Build history of the part. All positions in model axes, mm. A direction names the side the tool comes from. Give positions to 0.01 mm unless a question says otherwise; leave off trailing zeros. Write each loop counter-clockwise with the first axis right and the second up, starting at its lowest first coordinate (ties: lowest second). Pieces come first, ordered by that corner, then holes. Notation, with made-up numbers: M 85.5,-22.5 L 89.5,-22.5 A11 ccw 89.5,-13.5 Z; hole C -19,56 d1. An arc over 180 degrees is marked long. One line per item, written item: value. Start each with the question number.
from build123d import *

# Parameters (mm, degrees)
F1_DEPTH       = 20
F2_D           = 8
F2_CBORE_D     = 12.5
F2_CBORE_DEPTH = 12.5
F3_D           = 8
F3_CBORE_D     = 12.5
F3_CBORE_DEPTH = 12.5


with BuildPart() as f1:
    # F0 (on Front) → F1 (new body)
    with BuildSketch(Plane.XZ):
        Polygon((197.0788455009, 58.5275515914), (-137.9211544991, 58.5275515914), (-137.9211544991, -121.4724484086), (-102.9211544991, -121.4724484086), (-102.9211544991, -1.4724484086), (-77.9211544991, -1.4724484086), (-77.9211544991, -121.4724484086), (-42.9211544991, -121.4724484086), (-42.9211544991, -1.4724484086), (-17.9211544991, -1.4724484086), (-17.9211544991, -121.4724484086), (17.0788455009, -121.4724484086), (17.0788455009, -1.4724484086), (42.0788455009, -1.4724484086), (42.0788455009, -121.4724484086), (77.0788455009, -121.4724484086), (77.0788455009, -1.4724484086), (102.0788455009, -1.4724484086), (102.0788455009, -121.4724484086), (137.0788455009, -121.4724484086), (137.0788455009, -1.4724484086), (162.0788455009, -1.4724484086), (162.0788455009, -121.4724484086), (197.0788455009, -121.4724484086), align=None)
    extrude(amount=F1_DEPTH)

    # F2 (through all)
    with Locations(Plane(origin=(0, 0, 0), x_dir=(1, 0, 0), z_dir=(0, 1, 0))):
        with Locations((-69.9211544991, -30.5275515914)):
            CounterBoreHole(F2_D / 2, F2_CBORE_D / 2, F2_CBORE_DEPTH)

    # F3 (through all)
    with Locations(Plane(origin=(0, 0, 0), x_dir=(1, 0, 0), z_dir=(0, 1, 0))):
        with Locations((60.0788455009, -30.5275515914)):
            CounterBoreHole(F3_D / 2, F3_CBORE_D / 2, F3_CBORE_DEPTH)


solid = f1.part
1) Band-saw the part on B-B (y = -4.25). List the corners of the cut face in (x, z), then the cut area to 3 significant figures.
2) Probe line 1 along X through (y, z) = (-18.5, -89); line 2 along Z through (x, y) = (82, -2.75); line 3 along Z through (x, y) = (56, -5.25). List the from-to ranges inside material, lowest first. Write a range as from..to.
3) Drop flat-ended pins along their axis: P1, Ø1, axis at x = 25.5, y = -5.5, coming from the -Z side; P2, Ø10.5, axis at x = 60.08, z = 30.53, coming from the +Y side. Give the stop position or say it passes through.
4) Band-saw the part on A-A (z = -46). List the corners of the cut face in (x, y), then the cut area to 3 significant figures.
5) Mould opens along X. For faces 1 (the face through (-61, -10, -121.472)), 2 (the face through (-137.921, -10, -30)), 3 (the face through (77.079, -10, -62)) say: released by +X, released by -X, zero draft, split by the parting line, or undercut.
6) Tool access for faces 4 (the face through (-121, -10, -121.472)), 5 (the face through (66.04, -6.16, 28.65)), 6 (the face through (-42.921, -10, -62)): list every direction of +Z, -Z, +X, -X, +Y, -Y with a clear straight run to the whole face (end or side of a thin tool).
7) Band-saw the part on C-C (x = 150.5). List the corners of the cut face in (y, z), then the cut area to 3 significant figures.
Model answer:
1. outline: M -137.92,-121.47 L -102.92,-121.47 L -102.92,-1.47 L -77.92,-1.47 L -77.92,-121.47 L -42.92,-121.47 L -42.92,-1.47 L -17.92,-1.47 L -17.92,-121.47 L 17.08,-121.47 L 17.08,-1.47 L 42.08,-1.47 L 42.08,-121.47 L 77.08,-121.47 L 77.08,-1.47 L 102.08,-1.47 L 102.08,-121.47 L 137.08,-121.47 L 137.08,-1.47 L 162.08,-1.47 L 162.08,-121.47 L 197.08,-121.47 L 197.08,58.53 L -137.92,58.53 Z; hole C -69.92,30.53 d12.5; hole C 60.08,30.53 d12.5
1. area: 45,100 mm²
2. line 1: x = -137.92..-102.92, -77.92..-42.92, -17.92..17.08, 42.08..77.08, 102.08..137.08, 162.08..197.08
2. line 2: z = -1.47..58.53
2. line 3: z = -121.47..25.79, 35.26..58.53
3. P1: stops at z = -1.47
3. P2: stops at y = -12.5
4. outline: M -137.92,-20 L -102.92,-20 L -102.92,0 L -137.92,0 Z; M -77.92,-20 L -42.92,-20 L -42.92,0 L -77.92,0 Z; M -17.92,-20 L 17.08,-20 L 17.08,0 L -17.92,0 Z; M 42.08,-20 L 77.08,-20 L 77.08,0 L 42.08,0 Z; M 102.08,-20 L 137.08,-20 L 137.08,0 L 102.08,0 Z; M 162.08,-20 L 197.08,-20 L 197.08,0 L 162.08,0 Z
4. area: 4,200 mm²
5. face 1: zero draft
5. face 2: released by -X
5. face 3: undercut
6. face 4: -Z, +X, -X, +Y, -Y
6. face 5: +Y
6. face 6: -Z, +Y, -Y
7. outline: M -20,-1.47 L 0,-1.47 L 0,58.53 L -20,58.53 Z
7. area: 1,200 mm²
